Geometry: final body of the model. Coordinates: model frame, mm. Face numbers are marked on the shaded views. A direction names the side the tool comes from. Coordinates: 2 decimals unless noted, no trailing zeros. Write each loop counter-clockwise with the first axis right and the second up, starting at its lowest first coordinate (ties: lowest second). Pieces come first, ordered by that corner, then holes. Notation, with made-up numbers: M 27.5,-7.75 L 72.5,-7.75 A18 ccw 72.5,27.25 Z; hole C 30.5,-22 d6. An arc over 180 degrees is marked long. Write item = value, one per line. Start each with the question number.
Item 1: Reachability of the marked faces 1, 2 and 3 from +Z, -Z, +X, -X, +Y, -Y: full face, straight path, thin tool, end or side. Return the list, or none.
Item 2: Ray query, L1, parallel to Y at x = 0, z = -24 (3 decimals); L2, parallel to Y at x = 0, z = 43; L3, parallel to Z at x = -19, y = -40. Return the intervals inside material, ascending. Write a range as [from, to].
Item 3: Section A-A on y = -63.5. Output: boundary loops of the cut face in (x, z) (3 decimals), plus the area to 3 significant figures.
Item 4: Section D-D on y = 110. Output: boundary loops of the cut face in (x, z).
Item 5: First-contact query: pin 1 Ø2 at (x, y) = (-7, 98.5) entering from -Z; pin 2 Ø1.5 at (x, y) = (-57, 36) entering from -Z; pin 3 Ø4 at (x, y) = (2.5, -62.5) entering from +Z. Flat tips, straight axial feed; report the tip coordinate or a pass-through.
Item 6: Section B-B on z = 12. Output: boundary loops of the cut face in (x, y) (3 decimals), plus the area to 3 significant figures.
Item 7: Section C-C on x = 0. Output: boundary loops of the cut face in (y, z) (3 decimals), plus the area to 3 significant figures.
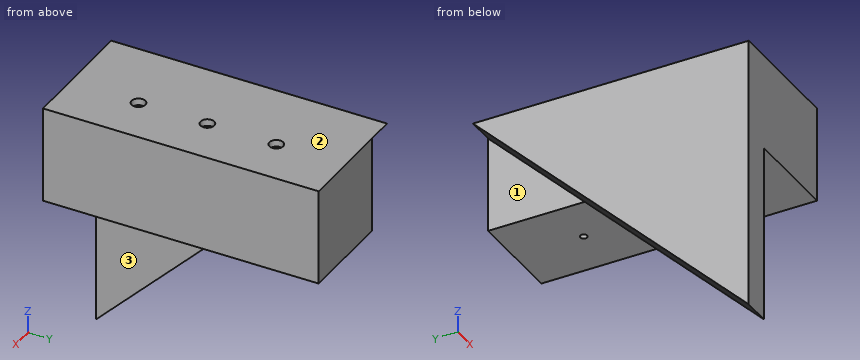
from build123d import *

# Parameters (mm, degrees)
F0_W           = 88.9
F0_H           = 88.9
F1_DEPTH       = 127
F3_D           = 6.35
F3_CBORE_D     = 12.7
F3_CBORE_DEPTH = 6.35
F6_DEPTH       = 25.4


with BuildPart() as f1:
    # F0 (on Front) → F1 (new body, symmetric)
    with BuildSketch(Plane.XZ):
        Rectangle(F0_W, F0_H)
    extrude(amount=F1_DEPTH, both=True)

    # F3 (through all)
    with Locations(Plane.XY.offset(44.45)):
        with Locations((0, 63.5), (0, 0), (0, -63.5)):
            CounterBoreHole(F3_D / 2, F3_CBORE_D / 2, F3_CBORE_DEPTH)

    # F5 (on face) → F6 (join)
    with BuildSketch(Plane(origin=(-44.45, 0, 0), x_dir=(0, -1, 0), z_dir=(-1, 0, 0))):
        Polygon((127, 44.45), (-127, 44.45), (127, -209.55), align=None)
    extrude(amount=F6_DEPTH)


solid = f1.part
Responses:
q1.face_1 = -Z, -X, +Y
q1.face_2 = +Z, +X, -X, +Y, -Y
q1.face_3 = -Z, +X, +Y, -Y
q2.L1 = [-127, -66.675], [-60.325, -3.175], [3.175, 60.325], [66.675, 127]
q2.L2 = [-127, -69.85], [-57.15, -6.35], [6.35, 57.15], [69.85, 127]
q2.L3 = [-44.45, 44.45]
q3.outline = M -69.85,-146.05 L -44.45,-146.05 L -44.45,-44.45 L -3.175,-44.45 L -3.175,38.1 L -6.35,38.1 L -6.35,44.45 L -69.85,44.45 Z; M 3.175,-44.45 L 44.45,-44.45 L 44.45,44.45 L 6.35,44.45 L 6.35,38.1 L 3.175,38.1 Z
q3.area = 12,100 mm²
q4.outline = M -69.85,27.45 L -44.45,27.45 L -44.45,-44.45 L 44.45,-44.45 L 44.45,44.45 L -69.85,44.45 Z
q5.pin_1 = -44.45
q5.pin_2 = -47.3
q5.pin_3 = 38.1
q6.outline = M -69.85,-127 L 44.45,-127 L 44.45,127 L -44.45,127 L -44.45,94.55 L -69.85,94.55 Z; hole C 0,-63.5 d6.35; hole C 0,0 d6.35; hole C 0,63.5 d6.35
q6.area = 28,100 mm²
q7.outline = M -127,-44.45 L -66.675,-44.45 L -66.675,38.1 L -69.85,38.1 L -69.85,44.45 L -127,44.45 Z; M -60.325,-44.45 L -3.175,-44.45 L -3.175,38.1 L -6.35,38.1 L -6.35,44.45 L -57.15,44.45 L -57.15,38.1 L -60.325,38.1 Z; M 3.175,-44.45 L 60.325,-44.45 L 60.325,38.1 L 57.15,38.1 L 57.15,44.45 L 6.35,44.45 L 6.35,38.1 L 3.175,38.1 Z; M 66.675,-44.45 L 127,-44.45 L 127,44.45 L 69.85,44.45 L 69.85,38.1 L 66.675,38.1 Z
q7.area = 20,800 mm²
